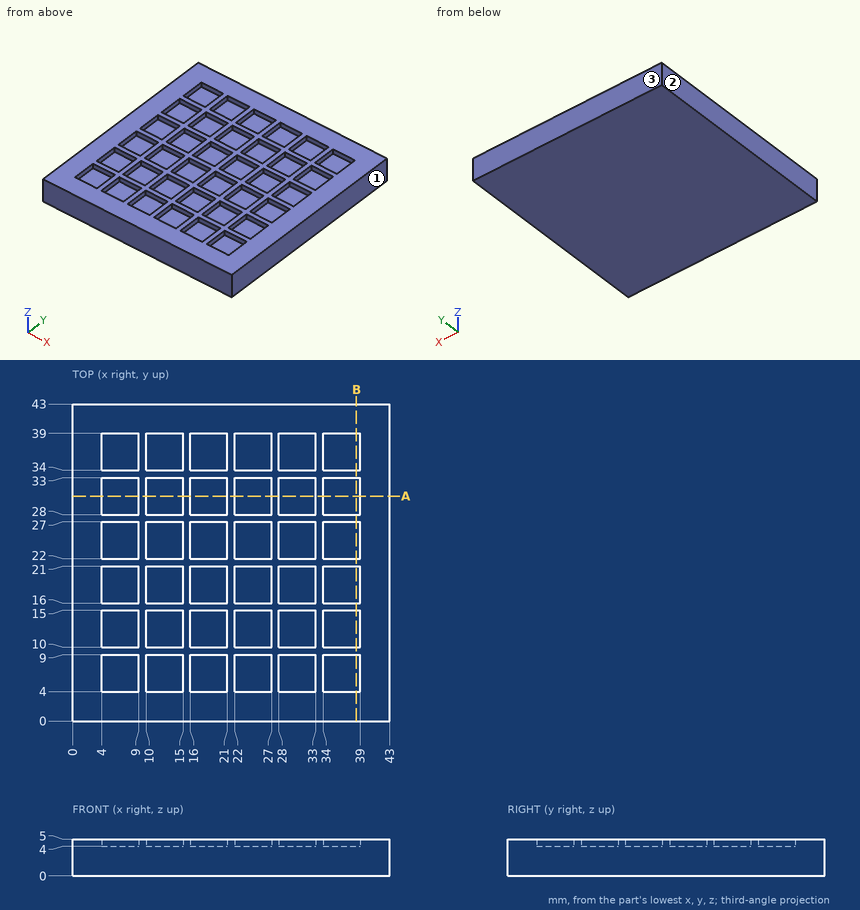
Check sheet for the drawn part. Datum: minimum x, y, z corner. Units: mm. Coordinates: 2 decimals unless noted, no trailing zeros. Order: outer loops, then holes, each group sorted by start corner. A loop starts at its lowest first (then second) coordinate and runs counter-clockwise, first axis right, second up. Notation, with made-up numbers: M -8,40.5 L 23,40.5 A23 cw 23,60.5 Z; hole C 22.5,36.5 d10. An arc over 180 degrees is marked long. One line per item, written item: value. Start each with the question number.
Item 1: Gauge pin test, flat ends, axial feed: pin 1 (0.8 mm diameter, centred on y = 18, z = 4.5, fed in from -X); pin 2 (1.5 mm diameter, centred on x = 12.5, y = 5.5, fed in from +Z). Record the tip position at first contact, or that the pin passes through.
Item 2: Mould release check, pull along X, two halves, no side actions. Record for the marked faces 1, 2 and 3: released by +X, released by -X, zero draft, split by the parting line, or undercut.
Item 3: Sectioned sample at A-A (y = 30.5). Enter the section's corners in (x, z).
Item 4: Scan line: probe 1 along Z at (x, y) = (5, 26). Record every from-to range of solid material in increasing order.
Conclusion:
1. pin 1: stops at x = 0
1. pin 2: stops at z = 4
2. face 1: released by +X
2. face 2: released by -X
2. face 3: zero draft
3. outline: M 0,0 L 43,0 L 43,5 L 39,5 L 39,4 L 34,4 L 34,5 L 33,5 L 33,4 L 28,4 L 28,5 L 27,5 L 27,4 L 22,4 L 22,5 L 21,5 L 21,4 L 16,4 L 16,5 L 15,5 L 15,4 L 10,4 L 10,5 L 9,5 L 9,4 L 4,4 L 4,5 L 0,5 Z
4. probe 1: z = 0 to 4
